Autodesk Inventor part; units mm, degrees
ref_plane "YZ Plane" through (0, 0, 0) normal (1, 0, 0) x (0, 1, 0)
ref_plane "XZ Plane" through (0, 0, 0) normal (0, 1, 0) x (-1, 0, 0)
ref_plane "XY Plane" through (0, 0, 0) normal (0, 0, 1) x (1, 0, 0)
sketch "Sketch2" plane through (0, 0, 0) normal (0, 0, 1) x (1, 0, 0)
  line L0 (-6.5, -6.5) -> (6.5, -6.5)
  line L1 (6.5, -6.5) -> (6.5, 6.5)
  line L2 (6.5, 6.5) -> (-6.5, 6.5)
  line L3 (-6.5, 6.5) -> (-6.5, -6.5)
  line L4 (-6.5, -6.5) -> (6.5, 6.5) construction
  line L5 (6.5, -6.5) -> (-6.5, 6.5) construction
  line L6 (-5.25, -5.25) -> (5.25, -5.25)
  line L7 (5.25, -5.25) -> (5.25, 5.25)
  line L8 (5.25, 5.25) -> (-5.25, 5.25)
  line L9 (-5.25, 5.25) -> (-5.25, -5.25)
  line L10 (-5.25, -5.25) -> (5.25, 5.25) construction
  line L11 (5.25, -5.25) -> (-5.25, 5.25) construction
  line L12 (-5.75, 5.75) -> (5.75, 5.75)
  line L13 (5.75, 5.75) -> (5.75, -5.75)
  line L14 (5.75, -5.75) -> (-5.75, -5.75)
  line L15 (-5.75, -5.75) -> (-5.75, 5.75)
  line L16 (-3.5, -3.5) -> (3.5, -3.5)
  line L17 (3.5, -3.5) -> (3.5, 3.5)
  line L18 (3.5, 3.5) -> (-3.5, 3.5)
  line L19 (-3.5, 3.5) -> (-3.5, -3.5)
  line L20 (-3.5, -3.5) -> (3.5, 3.5) construction
  line L21 (3.5, -3.5) -> (-3.5, 3.5) construction
  point P0 (0, 0)
  dimension "d0" = 13
  dimension "d1" = 13
  dimension "d2" = 10.5
  dimension "d3" = 10.5
  dimension "d4" = 0.5
  dimension "d5" = 7
  dimension "d6" = 7
extrude "Extrusion1" add sketch "Sketch2" along normal blind 2.5 contours L3 L2 L1 L0
extrude "Extrusion2" add sketch "Sketch2" along normal blind 1 contours L9 L8 L7 L6 | L12 L13 L14 L15 | L19 L18 L17 L16
extrude "Extrusion3" cut sketch "Sketch2" along normal blind 1 contours L19 L18 L17 L16
fillet "Fillet1" radius 2 4 edges at (-3.5, 3.5, 0.5) (-3.5, -3.5, 0.5) (3.5, 3.5, 0.5) (3.5, -3.5, 0.5)
chamfer "Chamfer1" distance 1 angle 45 8 edges at (0, 3.5, 0) (-2.9142, 2.9142, 0) (-3.5, 0, 0) (-2.9142, -2.9142, 0) (0, -3.5, 0) (2.9142, -2.9142, 0) (3.5, 0, 0) (2.9142, 2.9142, 0)
sketch "Sketch3" plane through (0, 0, 2.5) normal (0, 0, 1) x (1, 0, 0)
  line L0 (5.75, -5.75) -> (-5.75, -5.75)
  line L1 (-6.5, -6.5) -> (6.5, -6.5)
  line L2 (-5.75, -5.75) -> (5.75, -5.75)
  line L3 (5.75, -5.75) -> (5.75, -6.5)
  line L4 (5.75, -6.5) -> (-5.75, -6.5)
  line L5 (-5.75, -6.5) -> (-5.75, -5.75)
  point P0 (0, 0)
  dimension "d17" = 11.5
extrude "Extrusion4" cut sketch "Sketch3" against normal blind 1
properties part number "Optical module_lid"
Build history of the part. All positions in model axes, mm. A direction names the side the tool comes from. Coordinates: 2 decimals unless noted, no trailing zeros. Write each loop counter-clockwise with the first axis right and the second up, starting at its lowest first coordinate (ties: lowest second). Pieces come first, ordered by that corner, then holes.
(1) Cut at A-A on z = 1.2. List the corners of the cut face in (x, y), and give its area (4 significant figures).
(2) Cut at D-D on x = 5.5. List the corners of the cut face in (y, z).
(3) 3-axis set-ups, long thin cutter, end or side, ignore diameter. For faces 4 (the flat face through (-1, 6, 2.5)), 5 (the conical face through (3.18, 3.21, 0.6)), 6 (the flat face through (-4, 0, 1)): which of +Z, -Z, +X, -X, +Y, -Y reach the whole face in a straight line?
(4) Drill centre lines: line 1 (X direction, y = 4.75, z = 1.75); line 2 (Z direction, x = 4.5, y = 3). Where is each one in solid material? Low to high.
(5) Mould opens along X. For faces 1 (the flat face through (6.5, 0, 1)), 2 (the flat face through (0, -6.5, 1)), 3 (the flat face through (0, 5.75, 2)) say: pulls with the +X half, pulls with the -X half, needs draft (parallel to the pull), parting line crosses it, or undercut.
(6) Pin check, flat tip, straight feed: pin 1 Ø3 at (x, y) = (3.5, -3) entering from +Z. Stop position of the tip, or through.
Working result:
1. outline: (-6.5, -6.5) - (6.5, -6.5) - (6.5, 6.5) - (-6.5, 6.5) - close; hole (-5.75, -5.75) - (5.75, -5.75) - (5.75, 5.75) - (-5.75, 5.75) - close
1. area: 36.75 mm2
2. outline: (-6.5, 0) - (6.5, 0) - (6.5, 2.5) - (5.75, 2.5) - (5.75, 1) - (-5.75, 1) - (-5.75, 1.5) - (-6.5, 1.5) - close
3. face 4: +Z, +X, -X, +Y, -Y
3. face 5: -Z
3. face 6: +Z
4. line 1: x = -6.5 to -5.75, 5.75 to 6.5
4. line 2: z = 0 to 1
5. face 1: pulls with the +X half
5. face 2: needs draft
5. face 3: undercut
6. pin 1: stops at z = 1
